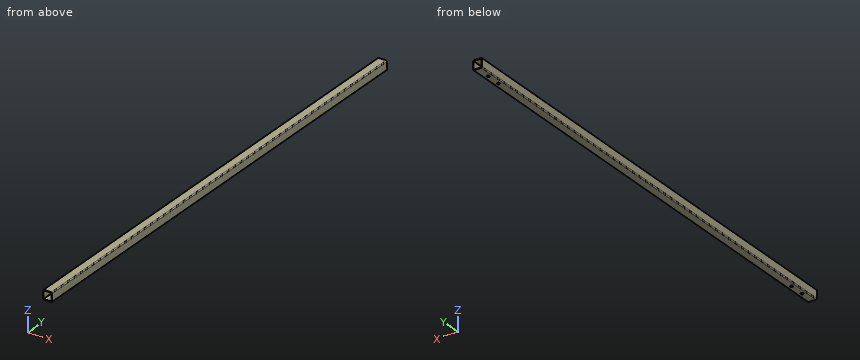
Autodesk Inventor part; units mm, degrees
ref_plane "XZ Plane" through (0, 0, 0) normal (0, 1, 0) x (-1, 0, 0)
sketch "Sketch1" plane through (0, 0, 0) normal (0, 1, 0) x (-1, 0, 0)
  line L0 (-12, 14) -> (12, 14) construction
  line L1 (14, 12) -> (14, -12) construction
  line L2 (12, -14) -> (-12, -14) construction
  line L3 (-14, -12) -> (-14, 12) construction
  line L4 (-14, 14) -> (14, -14) construction
  line L5 (14, 14) -> (-14, -14) construction
  arc A0 (14, 12) -> (12, 14) centre (12, 12) ccw construction
  arc A1 (12, -14) -> (14, -12) centre (12, -12) ccw construction
  arc A2 (-14, -12) -> (-12, -14) centre (-12, -12) ccw construction
  arc A3 (-12, 14) -> (-14, 12) centre (-12, 12) ccw construction
  line L6 (-12, -15) -> (12, -15)
  arc A4 (12, -15) -> (15, -12) centre (12, -12) ccw
  line L7 (15, -12) -> (15, 12)
  arc A5 (15, 12) -> (12, 15) centre (12, 12) ccw
  line L8 (12, 15) -> (-12, 15)
  arc A6 (-12, 15) -> (-15, 12) centre (-12, 12) ccw
  line L9 (-15, 12) -> (-15, -12)
  arc A7 (-15, -12) -> (-12, -15) centre (-12, -12) ccw
  line L10 (13, -12) -> (13, 12)
  arc A8 (13, 12) -> (12, 13) centre (12, 12) ccw
  line L11 (12, 13) -> (-12, 13)
  arc A9 (-12, 13) -> (-13, 12) centre (-12, 12) ccw
  line L12 (-13, 12) -> (-13, -12)
  arc A10 (-13, -12) -> (-12, -13) centre (-12, -12) ccw
  line L13 (-12, -13) -> (12, -13)
  arc A11 (12, -13) -> (13, -12) centre (12, -12) ccw
  point P0 (0, 0)
  point P1 (0, 0)
  point P2 (0, 0)
  dimension "d10" = 2
  dimension "depth" = 30
  dimension "width" = 30
  dimension "thickness" = 2
extrude "Extrusion1" add sketch "Sketch1" along normal blind 1600
sketch "Sketch2" plane through (12, 0, -15) normal (0, 0, -1) x (-1, 0, 0)
  line L0 (12, -390) -> (12, 2340) construction
  line L1 (0, 0) -> (24, 0)
  line L2 (0, 1600) -> (24, 1600)
  point P0 (12, 0)
  point P1 (12, 50)
  point P2 (12, 100)
  point P3 (12, 1550)
  point P4 (12, 1500)
  dimension "d16" = 50
  dimension "d17" = 50
  dimension "d18" = 50
  dimension "d20" = 50
hole "Hole1" at (0, 50, -15) at (0, 100, -15) at (0, 1550, -15) at (0, 1500, -15) direction (0, 0, 1) diameter 9 depth 20.2 tip angle 118
equation "\"d10\" = thickness"
properties part number "Przedluzka L1500" material "Steel"
Build history of the part. All positions in model axes, mm. Round coordinates to 2 decimals unless told otherwise and drop trailing zeros. Write each loop counter-clockwise with the first axis right and the second up, starting at its lowest first coordinate (ties: lowest second). Pieces come first, ordered by that corner, then holes. Notation, with made-up numbers: (6.5, 3) -> (52.5, 3) arc R7 ccw to (52.5, 13) -> close; hole circle Ø7 at (1, 63.25). An arc over 180 degrees is marked (long way). Put each result on its own line as item: value.
Item 1: Slice it at A-A, the plane z = -0.5. Give the cut face in (x, y).
Here are the results:
outline: (-15, 0) -> (-13, 0) -> (-13, 1600) -> (-15, 1600) -> close; (13, 0) -> (15, 0) -> (15, 1600) -> (13, 1600) -> close
Item 2: Flat gauge pins, fed straight in: P1, Ø5, axis at x = -9, z = -1.5, coming from the -Y side; P2, Ø7, axis at x = 0, y = 1500, coming from the -Z side. Where does each tip first touch, or does it go through?
Here are the results:
P1: passes through
P2: stops at z = 13
Item 3: Wall check: probe 1 along Y at (x, z) = (0, -14.2); probe 2 along Z at (x, y) = (-8.5, 245). Give the ranges that are in metal, low to high. Write a range as from..to.
Here are the results:
probe 1: y = 0..45.5, 54.5..95.5, 104.5..1495.5, 1504.5..1545.5, 1554.5..1600
probe 2: z = -15..-13, 13..15
Item 4: Slice it at B-B, the plane y = 1101. Give the cut face in (x, z).
Here are the results:
outline: (-15, -12) arc R3 ccw to (-12, -15) -> (12, -15) arc R3 ccw to (15, -12) -> (15, 12) arc R3 ccw to (12, 15) -> (-12, 15) arc R3 ccw to (-15, 12) -> close; hole (-13, -12) arc R1 ccw to (-12, -13) -> (12, -13) arc R1 ccw to (13, -12) -> (13, 12) arc R1 ccw to (12, 13) -> (-12, 13) arc R1 ccw to (-13, 12) -> close
